The drawing under review shows one solid part. Ordinate dimensions are in mm from its lowest x, y, z. A direction names the side the tool comes from. Round coordinates to 2 decimals unless told otherwise and drop trailing zeros. Write each loop counter-clockwise with the first axis right and the second up, starting at its lowest first coordinate (ties: lowest second). Pieces come first, ordered by that corner, then holes.
Item 1: To check wall thickness, follow L1, parallel to X at y = 9.5, z = 23.5; L2, parallel to Z at x = 22, y = 7; L3, parallel to Z at x = 22.5, y = 7.7 (3 decimals). State the ranges of each line that lie inside material, in increasing order.
Item 2: Draft analysis for pull direction X (two halves, no side actions). For the marked faces 4, 5 and 6, state which applies: +X half, -X half, draft (parallel to the pull), parting line (faces both ways), or undercut.
Item 3: Clearance check with flat-ended pins moving along their axes: pin 1 Ø1.5 at (y, z) = (1.5, 26) entering from -X; pin 2 Ø1 at (x, y) = (40, 3.5) entering from -Z; pin 3 Ø4 at (y, z) = (5, 22) entering from -X. State where each tip first meets the part, or that it passes through.
Item 4: Add section B-B (x = 22.5). Give the boundary of the cut face in (y, z).
Item 5: Machinability: for the marked faces 1, 2 and 3, which of the approach directions +Z, -Z, +X, -X, +Y, -Y give a long, thin tool a straight path to every point of the face, cutting with its end or side? Answer none if there is none.
Item 6: Add section A-A (y = 7). Give the boundary of the cut face in (x, z).
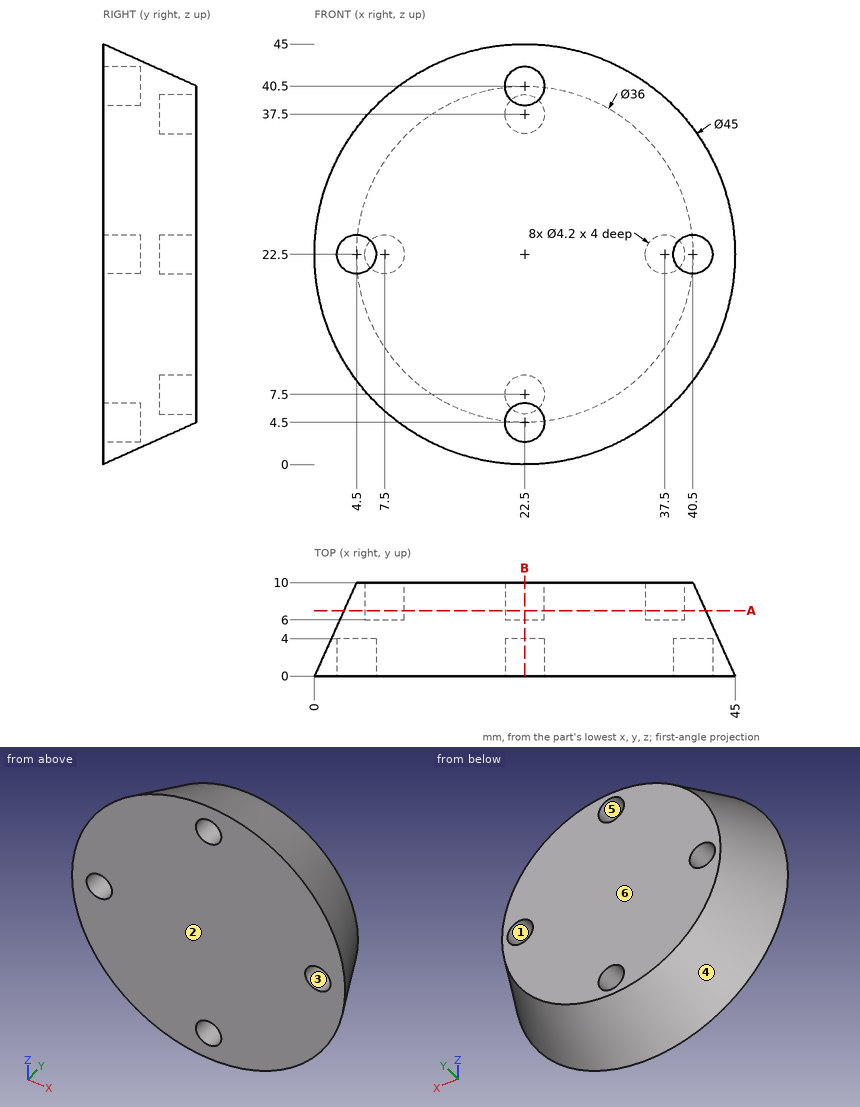
Numbers:
1. L1: x = 4.3 to 5.65, 9.35 to 35.65, 39.35 to 40.7
1. L2: z = 3.16 to 5.46, 9.54 to 35.46, 39.54 to 41.84
1. L3: z = 3.465 to 5.4, 9.6 to 35.4, 39.6 to 41.535
2. face 4: parting line
2. face 5: undercut
2. face 6: draft
3. pin 1: stops at x = 0.6
3. pin 2: stops at z = 10.2
3. pin 3: stops at x = 1.35
4. outline: (0, 0) - (10, 4.5) - (10, 5.4) - (6, 5.4) - (6, 9.6) - (10, 9.6) - (10, 35.4) - (6, 35.4) - (6, 39.6) - (10, 39.6) - (10, 40.5) - (0, 45) - (0, 42.6) - (4, 42.6) - (4, 38.4) - (0, 38.4) - (0, 6.6) - (4, 6.6) - (4, 2.4) - (0, 2.4) - close
5. face 1: +Y
5. face 2: +Z, -Z, +X, -X, -Y
5. face 3: -Y
6. outline: circle Ø38.7 at (22.5, 22.5); hole circle Ø4.2 at (7.5, 22.5); hole circle Ø4.2 at (22.5, 7.5); hole circle Ø4.2 at (22.5, 37.5); hole circle Ø4.2 at (37.5, 22.5)
